Part print with two shaded views. Sizes in mm from the minimum x, y, z corner. Round coordinates to 2 decimals unless told otherwise and drop trailing zeros. Loops run counter-clockwise (first coordinate to the right, second up) from the corner with the lowest first, then second, coordinate; pieces in that order, holes last. Notation, with made-up numbers: (39.25, 69.25) -> (81.25, 69.25) arc R26 ccw to (81.25, 104.25) -> close; hole circle Ø4 at (56, 9.5). An arc over 180 degrees is marked (long way). Answer as a JSON object with one key per item and string values. Group by question number.
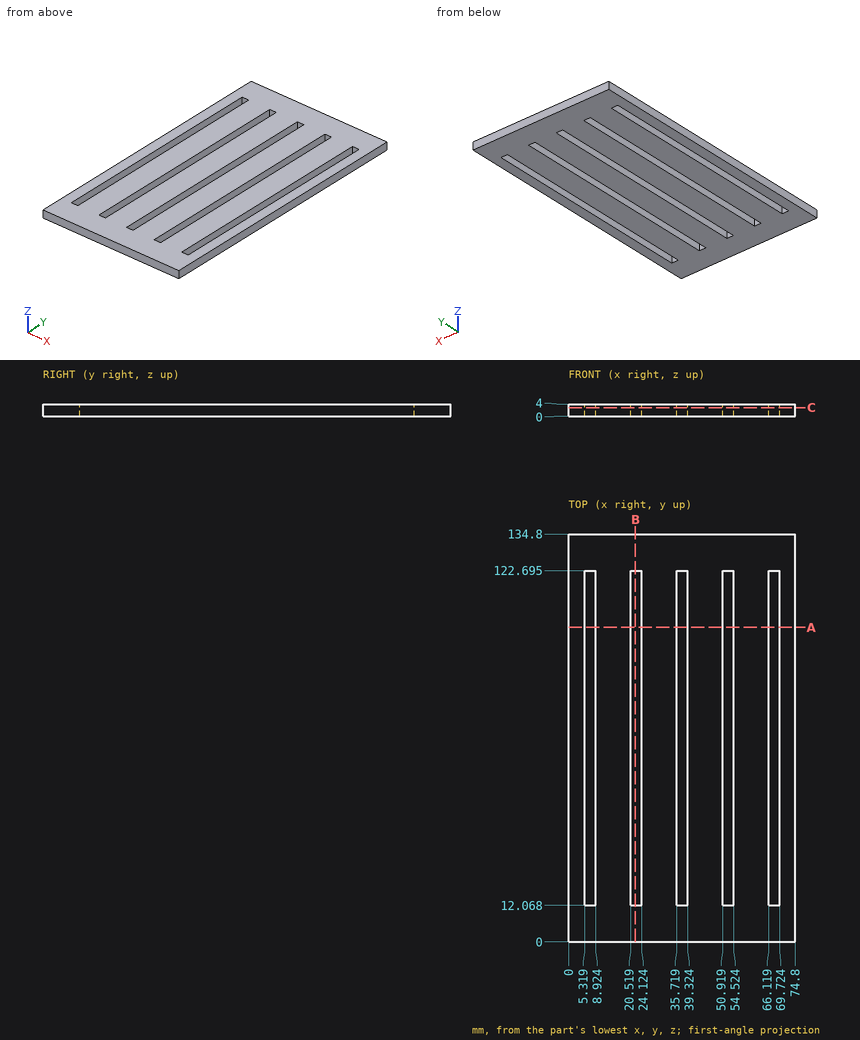
Item 1: Band-saw the part on C-C, the plane z = 2.8. List the corners of the cut face in (x, y) (1 decimal).
Item 2: Band-saw the part on A-A, the plane y = 104. List the corners of the cut face in (x, z) (1 decimal).
Item 3: Band-saw the part on B-B, the plane x = 22. List the corners of the cut face in (y, z) (1 decimal).
Item 4: Drill centre lines: line 1 (X direction, y = 82.5, z = 2.1) (1 decimal); line 2 (Y direction, x = 52.5, z = 0.3) (1 decimal). Where is each one in solid material? Low to high.
Entries:
{
 "1": {"outline": "(0, 0) -> (74.8, 0) -> (74.8, 134.8) -> (0, 134.8) -> close; hole (5.3, 12.1) -> (8.9, 12.1) -> (8.9, 122.7) -> (5.3, 122.7) -> close; hole (20.5, 12.1) -> (24.1, 12.1) -> (24.1, 122.7) -> (20.5, 122.7) -> close; hole (35.7, 12.1) -> (39.3, 12.1) -> (39.3, 122.7) -> (35.7, 122.7) -> close; hole (50.9, 12.1) -> (54.5, 12.1) -> (54.5, 122.7) -> (50.9, 122.7) -> close; hole (66.1, 12.1) -> (69.7, 12.1) -> (69.7, 122.7) -> (66.1, 122.7) -> close"},
 "2": {"outline": "(0, 0) -> (5.3, 0) -> (5.3, 4) -> (0, 4) -> close; (8.9, 0) -> (20.5, 0) -> (20.5, 4) -> (8.9, 4) -> close; (24.1, 0) -> (35.7, 0) -> (35.7, 4) -> (24.1, 4) -> close; (39.3, 0) -> (50.9, 0) -> (50.9, 4) -> (39.3, 4) -> close; (54.5, 0) -> (66.1, 0) -> (66.1, 4) -> (54.5, 4) -> close; (69.7, 0) -> (74.8, 0) -> (74.8, 4) -> (69.7, 4) -> close"},
 "3": {"outline": "(0, 0) -> (12.1, 0) -> (12.1, 4) -> (0, 4) -> close; (122.7, 0) -> (134.8, 0) -> (134.8, 4) -> (122.7, 4) -> close"},
 "4": {"line 1": "0 to 5.3, 8.9 to 20.5, 24.1 to 35.7, 39.3 to 50.9, 54.5 to 66.1, 69.7 to 74.8", "line 2": "0 to 12.1, 122.7 to 134.8"}
}
